```python
from build123d import *

# Parameters (mm, degrees)
F2_T     = -6.35
F4_R     = 28.3085495975
F5_DEPTH = 38.1
F6_R     = 6.35


with BuildPart() as f1:
    # F0 (on Front) → F1 (revolve)
    with BuildSketch(Plane.XZ):
        with BuildLine():
            Line((0, 0), (0, 50.0989693034))
            ThreePointArc((0, 50.0989693034), (-35.4253209249, 35.4253209249), (-50.0989693034, 0))
            Line((-50.0989693034, 0), (0, 0))
        make_face()
    revolve(axis=Axis((0, 0, 10.1562657768), (0, 0, -1)))

    # F2
    f2_openings = [f1.faces().sort_by_distance(p)[0] for p in [
        (0, 0, 0),
    ]]
    offset(amount=F2_T, openings=f2_openings)

    # F4 (on offset) → F5 (cut, symmetric)
    with BuildSketch(Plane.XY.offset(41.275)):
        Circle(F4_R)
    extrude(amount=F5_DEPTH, both=True, mode=Mode.SUBTRACT)

    # F6
    f6_edges = [f1.edges().sort_by_distance(p)[0] for p in [
        (0, -28.30855, 33.355634),
        (0, 28.30855, 33.355634),
    ]]
    fillet(f6_edges, radius=F6_R)


solid = f1.part
```
The model under review builds one solid part; all positions refer to its coordinate system, in mm. Give positions to 0.01 mm unless a question says otherwise; leave off trailing zeros. Write each loop counter-clockwise with the first axis right and the second up, starting at its lowest first coordinate (ties: lowest second). Pieces come first, ordered by that corner, then holes. Notation, with made-up numbers: (53.25, 79.5) - (104.25, 79.5) arc R19 cw to (104.25, 92.5) - close; hole circle Ø11 at (-24.5, 6.25). An arc over 180 degrees is marked (long way). Answer in a Markdown table with one row per item. Add a question column.
1. We need section B-B on y = -31.5. Write out the cut boundary in (x, z), then the cut area to 3 significant figures.
2. Draft analysis for pull direction X (two halves, no side actions). For faces 1 (the cylindrical face through (-22.46, -17.23, 38.79)), 2 (the flat face through (0, -44, 0)), state which applies: +X half, -X half, draft (parallel to the pull), parting line (faces both ways), or undercut.
3. Wall thickness on line 1 along X through (y, z) = (0, 37.3); line 2 along X through (y, z) = (34.5, 14); line 3 along Y through (x, z) = (-7, 23): over which ranges is each line inside the solid? List them lowest first. Write a range as [from, to].
4. Insertion check: P1, Ø1, axis at x = 19.5, z = 29, coming from the -Y side; P2, Ø1.5, axis at x = -9, z = 35.5, coming from the -Y side; P3, Ø1, axis at x = 38, y = 19, coming from the +Z side. Each pin has a flat end and moves straight along its axis. Give the tip position at first contact, or say it passes through.
5. We need section A-A on z = 38. Write out the cut boundary in (x, y).
6. We need section C-C on z = 13. Write out the cut boundary in (x, y), then the cut area to 3 significant figures.
Ans:
| question | item | result |
|---|---|---|
| 1 | outline | (-38.96, 0) - (-30.36, 0) arc R30.36 cw to (30.36, 0) - (38.96, 0) arc R38.96 ccw to start |
| 1 | area | 936 mm^2 |
| 2 | face 1 | undercut |
| 2 | face 2 | draft |
| 3 | line 1 | x = [-33.45, -28.31], [28.31, 33.45] |
| 3 | line 2 | x = [-33.52, -22.97], [22.97, 33.52] |
| 3 | line 3 | y = [-43.95, -36.55], [36.55, 43.95] |
| 4 | P1 | stops at y = -36.38 |
| 4 | P2 | stops at y = -34.97 |
| 4 | P3 | stops at z = 27.33 |
| 5 | outline | circle Ø65.3 at (0, 0); hole circle Ø56.62 at (0, 0) |
| 6 | outline | circle Ø96.77 at (0, 0); hole circle Ø83.55 at (0, 0) |
| 6 | area | 1,870 mm^2 |
